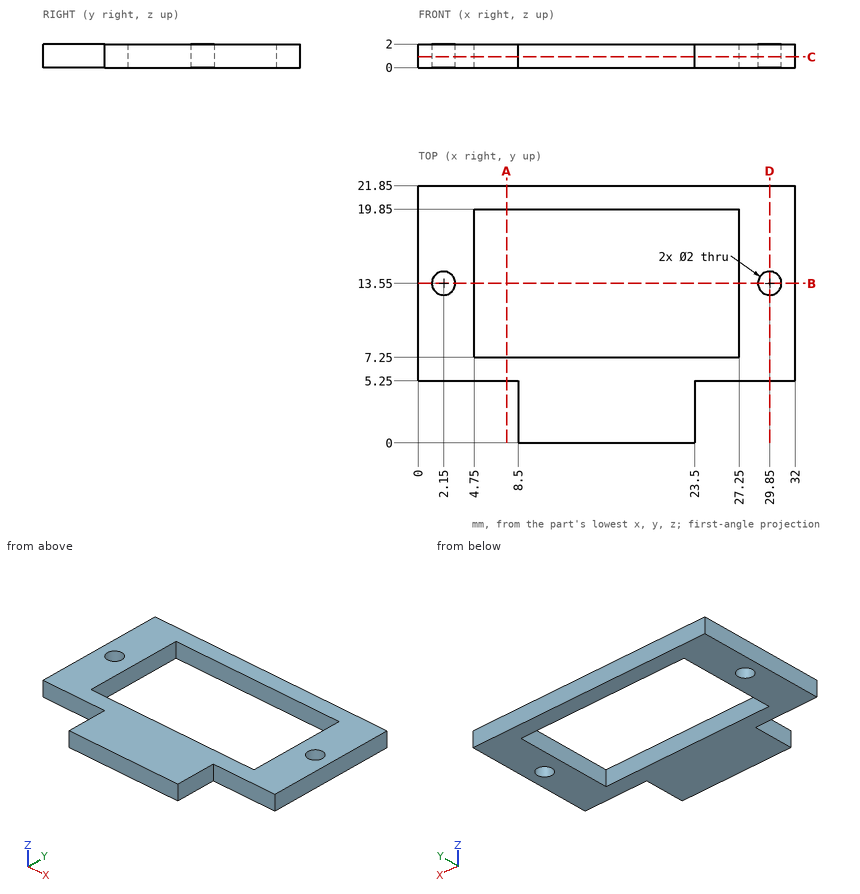
Print and shaded views of the part. All mm, measured from the part's lowest x, y and z. Give positions to 0.01 mm unless a question says otherwise; leave off trailing zeros. Loops run counter-clockwise (first coordinate to the right, second up) from the corner with the lowest first, then second, coordinate; pieces in that order, holes last. Notation, with made-up numbers: M 1.5,20 L 12.5,20 A5 cw 12.5,26 Z; hole C 72.25,16 d11. An arc over 180 degrees is marked long. Write each question's results on one line, items separated by ' | '.
Q1. Band-saw the part on C-C on z = 0.9. Write the cut outline in (x, y), and give its area (3 significant figures).
Geometry check:
outline: M 0,5.25 L 8.5,5.25 L 8.5,0 L 23.5,0 L 23.5,5.25 L 32,5.25 L 32,21.85 L 0,21.85 Z; hole C 2.15,13.55 d2; hole M 4.75,7.25 L 27.25,7.25 L 27.25,19.85 L 4.75,19.85 Z; hole C 29.85,13.55 d2 | area: 320 mm²
Q2. Flat gauge pins, fed straight in: P1, Ø1, axis at x = 3, z = 1.5, coming from the -Y side; P2, Ø1, axis at y = 4.5, z = 1.5, coming from the +X side; P3, Ø0.6, axis at y = 4, z = 0.5, coming from the -X side. Where does each tip first touch, or does it go through?
Geometry check:
P1: stops at y = 5.25 | P2: stops at x = 23.5 | P3: stops at x = 8.5
Q3. Band-saw the part on D-D on x = 29.85. Write the cut outline in (y, z).
Geometry check:
outline: M 5.25,0 L 12.55,0 L 12.55,2 L 5.25,2 Z; M 14.55,0 L 21.85,0 L 21.85,2 L 14.55,2 Z
Q4. Probe probe 1 along Y at (x, z) = (11, 1.5); probe 2 along X at (y, z) = (15.25, 0.35); probe 3 along Y at (x, z) = (7, 1.05). List the from-to ranges inside material, lowest first.
Geometry check:
probe 1: y = 0 to 7.25, 19.85 to 21.85 | probe 2: x = 0 to 4.75, 27.25 to 32 | probe 3: y = 5.25 to 7.25, 19.85 to 21.85
Q5. Band-saw the part on A-A on x = 7.5. Write the cut outline in (y, z).
Geometry check:
outline: M 5.25,0 L 7.25,0 L 7.25,2 L 5.25,2 Z; M 19.85,0 L 21.85,0 L 21.85,2 L 19.85,2 Z
Q6. Band-saw the part on B-B on y = 13.55. Write the cut outline in (x, z).
Geometry check:
outline: M 0,0 L 1.15,0 L 1.15,2 L 0,2 Z; M 3.15,0 L 4.75,0 L 4.75,2 L 3.15,2 Z; M 27.25,0 L 28.85,0 L 28.85,2 L 27.25,2 Z; M 30.85,0 L 32,0 L 32,2 L 30.85,2 Z
